Autodesk Fusion 360 part; units mm, degrees
sketch "Sketch1" plane through (0, 0, 0) normal (0, 0, 1) x (1, 0, 0)
  circle A0 centre (0, 0) radius 50
extrude "Extrude1" add sketch "Sketch1" along normal blind 70
sketch "Sketch2" plane through (0, 0, 0) normal (0, 0, -1) x (1, 0, 0)
  circle A0 centre (0, 0) radius 50
  circle A1 centre (0, 0) radius 40
  dimension "d3" = 80
extrude "Extrude2" cut sketch "Sketch2" against normal blind 10 contours A1
sketch "Sketch3" plane through (0, 0, 70) normal (0, 0, 1) x (-1, 0, 0)
  circle A0 centre (0, 0) radius 50
  circle A1 centre (0, 0) radius 46.5
  dimension "d6" = 93
extrude "Extrude3" cut sketch "Sketch3" against normal blind 2 contours A1
sketch "Sketch4" plane through (0, 0, 68) normal (0, 0, 1) x (-1, 0, 0)
  circle A0 centre (0, 0) radius 46.5
  circle A1 centre (0, 0) radius 43.5
  dimension "d9" = 87
extrude "Extrude4" cut sketch "Sketch4" against normal blind 50 contours A1
sketch "Sketch5" plane through (0, 0, 68) normal (0, 0, 1) x (-1, 0, 0)
  circle A0 centre (0, 0) radius 43.5
  circle A1 centre (0, 0) radius 46.5
  arc A2 (-2.5, -46.4327) -> (2.5, -46.4327) centre (0, 0) ccw
  arc A3 (2.5, 46.4327) -> (-2.5, 46.4327) centre (0, 0) ccw
  line L0 (2.5, 43.4281) -> (-2.5, 43.4281)
  line L1 (2.5, -43.4281) -> (-2.5, -43.4281)
  line L2 (2.5, -46.4327) -> (2.5, -43.4281)
  line L3 (2.5, 43.4281) -> (2.5, 46.4327)
  line L4 (-2.5, 46.4327) -> (-2.5, 43.4281)
  line L5 (-2.5, -43.4281) -> (-2.5, -46.4327)
  dimension "d12" = 5
extrude "Extrude5" cut sketch "Sketch5" against normal blind 15 contours A0 A1 A3 L3 L4 | A0 A1 A2 L2 L5
sketch "Sketch6" plane through (0, 0, 53) normal (0, 0, 1) x (-1, 0, 0)
  line L0 (2.5, 43.4281) -> (2.5, 46.4327)
  arc A0 (2.5, 46.4327) -> (-2.5, 46.4327) centre (0, 0) ccw
  line L1 (-2.5, 46.4327) -> (-2.5, 43.4281)
  arc A1 (2.5, 43.4281) -> (-2.5, 43.4281) centre (0, 0) ccw
  circle A2 centre (0, 0) radius 46.5
  line L2 (-2.5, 46.4327) -> (7.4711, -45.8959)
  line L3 (7.4711, -45.8959) -> (2.5, -46.4327)
  line L4 (2.5, -46.4327) -> (-7.4711, 45.8959)
  line L5 (-7.4711, 45.8959) -> (-2.5, 46.4327)
  dimension "d15" = 93
  dimension "d16" = 5
extrude "Extrude6" cut sketch "Sketch6" along normal blind 2 contours L1 A1 L2 L3 L4 L5
sketch "Sketch7" plane through (0, 0, 68) normal (0, 0, 1) x (-1, 0, 0)
  line L0 (-2.5, 43.4281) -> (-2.5, 46.4327)
  arc A0 (-2.5, 46.4327) -> (-2.5, -46.4327) centre (0, 0) ccw
  line L1 (-2.5, -46.4327) -> (-2.5, -43.4281)
  arc A1 (-2.5, 43.4281) -> (-2.5, -43.4281) centre (0, 0) ccw
  line L2 (-46.1113, 6) -> (-0.7807, 6)
  line L3 (-43.0404, -17.6004) -> (0.7807, -6)
  line L4 (43.0404, 17.6004) -> (-0.7807, 6)
  line L5 (46.1113, -6) -> (0.7807, -6)
  arc A2 (-46.1113, 6) -> (-43.0404, -17.6004) centre (0, 0) ccw
  arc A3 (46.1113, -6) -> (43.0404, 17.6004) centre (0, 0) ccw
  dimension "d19" = 93
  dimension "d20" = 12
  dimension "d21" = 12
extrude "Extrude7" cut sketch "Sketch7" against normal blind 50 contours A1 L2 L3 L4 L5 A3 | A0 A1 L2 L3 A2
sketch "Sketch8" plane through (0, 0, 18) normal (0, 0, 1) x (-1, 0, 0)
  arc A0 (40.1141, 16.8258) -> (-43.0842, 6) centre (0, 0) ccw
  line L0 (-43.0842, 6) -> (-46.1113, 6)
  arc A1 (-46.1113, 6) -> (-43.0404, -17.6004) centre (0, 0) ccw
  line L1 (-43.0404, -17.6004) -> (-40.1141, -16.8258)
  arc A2 (-40.1141, -16.8258) -> (43.0842, -6) centre (0, 0) ccw
  line L2 (43.0842, -6) -> (46.1113, -6)
  arc A3 (46.1113, -6) -> (43.0404, 17.6004) centre (0, 0) ccw
  line L3 (43.0404, 17.6004) -> (40.1141, 16.8258)
fillet "Fillet1" radius 2 1 edges at (-46.6164, -18.0808, 0)
sketch "Sketch11" plane through (0, 0, 68) normal (0, 0, 1) x (-1, 0, 0)
  line L0 (40.1141, 16.8258) -> (43.0404, 17.6004)
  arc A0 (43.0404, 17.6004) -> (2.5, 46.4327) centre (0, 0) ccw
  line L1 (2.5, 46.4327) -> (2.5, 43.4281)
  arc A1 (40.1141, 16.8258) -> (2.5, 43.4281) centre (0, 0) ccw
  line L2 (40.1141, 16.8258) -> (2.5, 43.4281)
  arc A2 (40.1141, 16.8258) -> (2.5, 43.4281) centre (0, 0) ccw
  dimension "d27" = 87
extrude "Extrude8" add sketch "Sketch11" against normal blind 50 contours A1 L2 A2
sketch "Sketch12" plane through (0, 0, 68) normal (0, 0, 1) x (-1, 0, 0)
  line L0 (40.1141, 16.8258) -> (43.0404, 17.6004)
  arc A0 (43.0404, 17.6004) -> (2.5, 46.4327) centre (0, 0) ccw
  line L1 (2.5, 46.4327) -> (2.5, 43.4281)
  line L2 (2.5, 43.4281) -> (40.1141, 16.8258)
  line L3 (40.1141, 16.8258) -> (46.4504, 18.5031)
  line L4 (2.5, 43.4281) -> (2.5, 49.9375)
  line L5 (46.4504, 18.5031) -> (2.5, 49.9375)
  arc A1 (46.4504, 18.5031) -> (2.5, 49.9375) centre (0, 0) ccw
  dimension "d30" = 100
extrude "Extrude9" cut sketch "Sketch12" against normal blind 30 from surface at -18 contours A0 L5 | A0 L5 A1
sketch "Sketch13" plane through (0, 0, 68) normal (0, 0, 1) x (-1, 0, 0)
  line L0 (40.1141, 16.8258) -> (43.0404, 17.6004)
  arc A0 (43.0404, 17.6004) -> (2.5, 46.4327) centre (0, 0) ccw
  line L1 (2.5, 46.4327) -> (2.5, 43.4281)
  line L2 (2.5, 43.4281) -> (40.1141, 16.8258)
  circle A1 centre (0, 0) radius 43.5
  line L3 (2.5, 43.4281) -> (40.1141, 16.8258)
extrude "Extrude10" cut sketch "Sketch13" against normal blind 15 contours L2 A1 L3 picked at (-1.1422, 13.8177)
sketch "Sketch14" plane through (0, 0, 0) normal (0, 0, -1) x (1, 0, 0)
  circle A0 centre (0, 0) radius 40
  circle A1 centre (0, 0) radius 48
  circle A2 centre (0, 0) radius 50
  dimension "d36" = 100
sketch "Sketch15" plane through (-24.4752, -34.2203, 0) normal (-0.5817, -0.8134, 0) x (0.8134, -0.5817, 0)
  line L0 (27.0174, 50) -> (-27.0174, 50)
  line L1 (-27.0174, 50) -> (-27.0174, 20)
  line L2 (-27.0174, 20) -> (27.0174, 20)
  line L3 (27.0174, 20) -> (27.0174, 50)
  line L4 (-27.0174, 20) -> (-27.0174, 0)
  line L5 (-27.0174, 0) -> (27.0174, 0)
  line L6 (27.0174, 0) -> (27.0174, 20)
sketch "Sketch16" plane through (0, 0, 0) normal (0, 0, -1) x (1, 0, 0)
  line L0 (-46.5152, 18.3394) -> (-2.261, 49.9489)
  line L1 (-2.261, 49.9489) -> (46.5152, -18.3394)
  line L2 (2.261, -49.9489) -> (-46.5152, 18.3394)
  circle A0 centre (0, 0) radius 50
  line L3 (46.5152, -18.3394) -> (29.7583, -30.3084)
  line L4 (19.0179, -37.9799) -> (2.261, -49.9489)
  line L5 (29.7583, -30.3084) -> (43.266, -49.2197)
  line L6 (43.266, -49.2197) -> (32.5257, -56.8912)
  line L7 (32.5257, -56.8912) -> (19.0179, -37.9799)
  line L8 (29.7583, -30.3084) -> (17.998, -13.8436)
  line L9 (17.998, -13.8436) -> (7.2576, -21.5151)
  line L10 (7.2576, -21.5151) -> (19.0179, -37.9799)
extrude "Extrude11" cut sketch "Sketch16" against normal blind 10 contours A0 L5 L7 L8 L9 L10 | A0 L5 L6 L7
fillet "Fillet2" radius 2 1 edges at (31.2391, 32.3815, 10)
fillet "Fillet3" radius 2 1 edges at (20.4987, 40.053, 10)
hole "Hole1" at (16.3478, 22.8843, 18) direction (0, 0, -1) diameter 15 depth 20 tip angle 118
sketch "Sketch18" plane through (-24.4752, -34.2203, 0) normal (-0.5817, -0.8134, 0) x (0.8134, -0.5817, 0)
  line L0 (27.0174, 50) -> (-27.0174, 50)
  line L1 (-27.0174, 50) -> (-27.0174, 20)
  line L2 (-27.0174, 20) -> (27.0174, 20)
  line L3 (27.0174, 20) -> (27.0174, 50)
  line L4 (-27.0174, 35) -> (27.0174, 35)
  line L5 (0, 35) -> (0, 20)
  line L6 (0, 27.5) -> (27.0174, 27.5)
  line L7 (13.5087, 27.5) -> (13.5087, 35)
  line L8 (0, 27.5) -> (-27.0174, 27.5)
  line L9 (-27.0174, 27.5) -> (-13.5087, 27.5)
  line L10 (-13.5087, 35) -> (-13.5087, 27.5)
  line L11 (0, 35) -> (0, 50)
  line L12 (0, 42.5) -> (27.0174, 42.5)
hole "Hole6" at (-35.4628, -26.3617, 27.5) direction (0.5817, 0.8134, 0) diameter 5 depth 10 tip angle 118
hole "Hole7" at (-13.4876, -42.0789, 27.5) direction (0.5817, 0.8134, 0) diameter 5 depth 10 tip angle 118
hole "Hole8" at (-24.4752, -34.2203, 35) direction (0.5817, 0.8134, 0) diameter 10 depth 10 tip angle 118
sketch "Sketch19" plane through (0, 0, 18) normal (0, 0, 1) x (-1, 0, 0)
  circle A0 centre (-16.3478, -22.8843) radius 7.5
  line L0 (40.1141, 16.8258) -> (2.5, 43.4281)
  arc A1 (2.5, 43.4281) -> (-43.0842, 6) centre (0, 0) ccw
  line L1 (-43.0842, 6) -> (-46.1113, 6)
  arc A2 (-46.1113, 6) -> (-43.0404, -17.6004) centre (0, 0) ccw
  line L2 (-43.0404, -17.6004) -> (-40.1141, -16.8258)
  arc A3 (-40.1141, -16.8258) -> (43.0842, -6) centre (0, 0) ccw
  line L3 (43.0842, -6) -> (46.1113, -6)
  arc A4 (46.1113, -6) -> (43.0404, 17.6004) centre (0, 0) ccw
  line L4 (43.0404, 17.6004) -> (40.1141, 16.8258)
  circle A5 centre (0, 0) radius 46.5
  circle A6 centre (0, 0) radius 46.5
  line L5 (43.0404, 17.6004) -> (-43.0404, -17.6004)
  line L6 (-46.1113, 6) -> (46.1113, -6)
hole "Hole9" at (0, 0, 18) direction (0, 0, -1) diameter 5 depth 8 tip angle 118
pattern_linear "R-Pattern1" count 2 spacing 10 along (0.8164, -0.5774, 0) of "Hole9"
pattern_linear "R-Pattern2" count 2 spacing 10 along (-0.8164, 0.5774, 0) of "Hole9"
The listing builds one solid part. Answer for the finished solid, in the listing's coordinates (mm). A direction names the side the tool comes from. Give positions to 0.01 mm unless a question says otherwise; leave off trailing zeros. Order: outer loops, then holes, each group sorted by start corner. A loop starts at its lowest first (then second) coordinate and runs counter-clockwise, first axis right, second up. Notation, with made-up numbers: (85, 85.5) - (138, 85.5) arc R22 cw to (138, 97.5) - close; hole circle Ø7 at (4, 9.25). An arc over 180 degrees is marked (long way). Use one line per item in the form item = value. Start each with the question number.
(1) A cutting plane is placed at A-A, the plane y = 0. Write down the section's boundary in (x, z), then the cut area to 3 significant figures.
(2) For faces 1 (the flat face through (3, -45, 53)), 2 (the flat face through (-1, -8, 10)), 3 (the flat face through (2.5, 45, 61)), determine the directions among +Z, -Z, +X, -X, +Y, -Y from which every point of the face is accessible in a straight line to the end or side of a thin tool.
(3) A cutting plane is placed at B-B, the plane z = 28. Write down the section's boundary in (x, y).
(4) Consider line 1 (Y direction, x = 0, z = 6); line 2 (Y direction, x = 0, z = 13.75). Determine where each line is inside the solid, lowest interval first. Write a range as from..to.
(5) The mould has two halves that part along X. Classify faces 4 (the flat face through (-26, -37, 50)), 5 (the cylindrical face through (-12.5, -39.5, 25.1)): released by +X, released by -X, zero draft, split by the parting line, or undercut.
(6) A cutting plane is placed at C-C, the plane x = 0. Write down the section's boundary in (y, z).
(7) Flat-ended cylindrical pins translate along their axes: pin 1 Ø1.5 at (y, z) = (-6.5, 51.5) entering from +X; pin 2 Ø12 at (x, z) = (-35.5, 56) entering from +Y; pin 3 Ø10 at (y, z) = (-39.5, 9) entering from -X. Find the tip coordinate at first contact, or state that the pin passes through.
Ans:
q1.outline = (-50, 2) arc R2 ccw to (-48, 0) - (-40, 0) - (-40, 10) - (-2.5, 10) - (-2.5, 18) - (-46.5, 18) - (-46.5, 70) - (-50, 70) - close; (2.5, 10) - (40, 10) - (40, 0) - (48, 0) arc R2 ccw to (50, 2) - (50, 70) - (46.5, 70) - (46.5, 18) - (2.5, 18) - close
q1.area = 1,320 mm^2
q2.face_1 = none
q2.face_2 = -Z
q2.face_3 = +Z
q3.outline = (-46.45, -18.5) - (-37.46, -24.94) - (-34.5, -20.8) - (-40.11, -16.83) - (-43.04, -17.6) arc R46.5 cw to (-46.11, 6) - (-43.08, 6) arc R43.5 cw to (40.11, 16.83) - (43.04, 17.6) arc R46.5 cw to (46.11, -6) - (43.08, -6) arc R43.5 cw to (-2.5, -43.43) - (-8.44, -39.23) - (-11.5, -43.5) - (-2.5, -49.94) arc R50 ccw (long way) to start; (-33.47, -27.79) - (-15.48, -40.65) - (-12.44, -36.4) - (-30.5, -23.63) - close
q4.line_1 = -50..-40, 40..50
q4.line_2 = -50..-2.5, 2.5..50
q5.face_4 = zero draft
q5.face_5 = undercut
q6.outline = (-50, 2) arc R2 ccw to (-48, 0) - (-40, 0) - (-40, 10) - (-2.5, 10) - (-2.5, 18) - (-43.5, 18) - (-43.5, 53) - (-46.5, 53) - (-46.5, 70) - (-50, 70) - close; (2.5, 10) - (40, 10) - (40, 0) - (48, 0) arc R2 ccw to (50, 2) - (50, 70) - (46.5, 70) - (46.5, 53) - (43.5, 53) - (43.5, 18) - (2.5, 18) - close
q7.pin_1 = 49.67
q7.pin_2 = 40.37
q7.pin_3 = -36.19
